Design review of the part built by this model. Coordinates are the model's own, in mm. Give positions to 0.01 mm unless a question says otherwise; leave off trailing zeros. Order: outer loops, then holes, each group sorted by start corner. A loop starts at its lowest first (then second) coordinate and runs counter-clockwise, first axis right, second up.
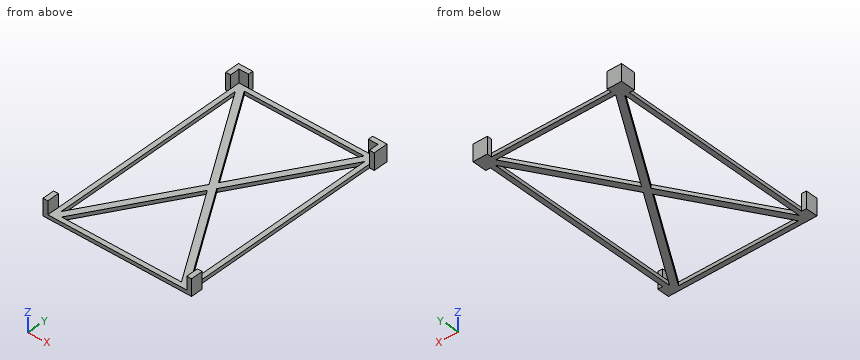
```python
from build123d import *

# Parameters (mm, degrees)
CROQUIS1_W              = 58
CROQUIS1_H              = 90
CROQUIS1_W_2            = 54
CROQUIS1_H_2            = 86
SALIENTE_EXTRUIR1_DEPTH = 1.5
CROQUIS2_W              = 2
CROQUIS2_H              = 5
SALIENTE_EXTRUIR2_DEPTH = 7
SALIENTE_EXTRUIR3_START = -1.5
SALIENTE_EXTRUIR3_DEPTH = 1.5


with BuildPart() as part:
    # Croquis1 → Saliente-Extruir1 (new body)
    with BuildSketch(Plane.XY):
        with Locations((-67.00177265, -15.055922694)):
            Rectangle(CROQUIS1_W, CROQUIS1_H)
        with Locations((-67.00177265, -15.055922694)):
            Rectangle(CROQUIS1_W_2, CROQUIS1_H_2, mode=Mode.SUBTRACT)
    extrude(amount=SALIENTE_EXTRUIR1_DEPTH)

    # Croquis2 → Saliente-Extruir2 (add)
    with BuildSketch(Plane(origin=(0, 0, 0), x_dir=(-1, 0, 0), z_dir=(0, 0, -1))):
        with Locations((37.00177265, -57.555922694)):
            Rectangle(CROQUIS2_W, CROQUIS2_H)
        Polygon((38.00177265, 29.944077306), (38.00177265, 25.944077306), (36.00177265, 25.944077306), (36.00177265, 31.944077306), (42.00177265, 31.944077306), (42.00177265, 29.944077306), align=None)
        Polygon((92.00177265, 29.944077306), (96.00177265, 29.944077306), (96.00177265, 25.944077306), (98.00177265, 25.944077306), (98.00177265, 31.944077306), (92.00177265, 31.944077306), align=None)
        with Locations((97.00177265, -57.555922694)):
            Rectangle(CROQUIS2_W, CROQUIS2_H)
    extrude(amount=-SALIENTE_EXTRUIR2_DEPTH)

    # Croquis3 → Saliente-Extruir3 (add)
    with BuildSketch(Plane(origin=(0, 0, 0), x_dir=(-1, 0, 0), z_dir=(0, 0, -1)).offset(SALIENTE_EXTRUIR3_START)):
        Polygon((94.00177265, -56.055922694), (68.620820269, -15.055922694), (94.00177265, 25.944077306), (94.00177265, 27.944077306), (92.00177265, 27.944077306), (67.00177265, -12.440538078), (42.00177265, 27.944077306), (40.00177265, 27.944077306), (40.00177265, 25.944077306), (65.382725031, -15.055922694), (40.00177265, -56.055922694), (40.00177265, -58.055922694), (42.00177265, -58.055922694), (67.00177265, -17.671307309), (92.00177265, -58.055922694), (94.00177265, -58.055922694), align=None)
    extrude(amount=SALIENTE_EXTRUIR3_DEPTH)


solid = part.part
```
1. Take a section at C-C (y = 9). State the section outline as (x, z) points, then the cut area to 3 significant figures.
Recorded:
outline: (-96, 0) - (-94, 0) - (-94, 1.5) - (-96, 1.5) - close; (-83.51, 0) - (-80.27, 0) - (-80.27, 1.5) - (-83.51, 1.5) - close; (-53.73, 0) - (-50.49, 0) - (-50.49, 1.5) - (-53.73, 1.5) - close; (-40, 0) - (-38, 0) - (-38, 1.5) - (-40, 1.5) - close
area: 15.7 mm2
2. For pin 1 (3 mm diameter, centred on x = -63, z = 3.5, fed in from -Y); pin 2 (4 mm diameter, centred on x = -53, y = -41, fed in from -Z); pin 3 (1.2 mm diameter, centred on x = -93.5, z = 5.5, fed in from -Y); pin 4 (1.2 mm diameter, centred on y = -13, z = 1, fed in from +X), all flat-tipped, find the tip position at first contact; note any pin that passes through.
Recorded:
pin 1: passes through
pin 2: stops at z = 0
pin 3: stops at y = 29.94
pin 4: stops at x = -38
3. Take a section at B-B (x = -59.5). State the section outline as (y, z) points, then the cut area to 3 significant figures.
Recorded:
outline: (-60.06, 0) - (-58.06, 0) - (-58.06, 1.5) - (-60.06, 1.5) - close; (-29.79, 0) - (-24.56, 0) - (-24.56, 1.5) - (-29.79, 1.5) - close; (-5.55, 0) - (-0.32, 0) - (-0.32, 1.5) - (-5.55, 1.5) - close; (27.94, 0) - (29.94, 0) - (29.94, 1.5) - (27.94, 1.5) - close
area: 21.7 mm2
4. For line 1 along Y through (x, z) = (-56, 0.5); line 2 along X through (y, z) = (-36.5, 1); line 3 along X through (y, z) = (-9.5, 0.5), list the stretches that pass through material, from the lowest coordinate up.
Recorded:
line 1: y = -60.06 to -58.06, -35.44 to -30.21, 0.1 to 5.33, 27.94 to 29.94
line 2: x = -96 to -94, -81.9 to -78.66, -55.35 to -52.11, -40 to -38
line 3: x = -96 to -94, -72.06 to -68.82, -65.18 to -61.94, -40 to -38
5. Take a section at A-A (z = 4.5). State the section outline as (x, y) points, then the cut area to 3 significant figures.
Recorded:
outline: (-98, -60.06) - (-96, -60.06) - (-96, -55.06) - (-98, -55.06) - close; (-98, 25.94) - (-96, 25.94) - (-96, 29.94) - (-92, 29.94) - (-92, 31.94) - (-98, 31.94) - close; (-42, 29.94) - (-38, 29.94) - (-38, 25.94) - (-36, 25.94) - (-36, 31.94) - (-42, 31.94) - close; (-38, -60.06) - (-36, -60.06) - (-36, -55.06) - (-38, -55.06) - close
area: 60.0 mm2
